Read the model definition and answer for the solid it produces. Units are mm, in the model's axes. A direction names the side the tool comes from. Give positions to 0.01 mm unless a question says otherwise; leave off trailing zeros. Write each loop counter-clockwise with the first axis right and the second up, starting at its lowest first coordinate (ties: lowest second). Pieces come first, ordered by that corner, then holes.
```python
from build123d import *

# Parameters (mm, degrees)
SKETCH_1_W          = 10
SKETCH_1_H          = 10
SKETCH_1_W_2        = 8
SKETCH_1_H_2        = 8
EXTRUDE_1_DEPTH     = 327
SKETCH_2_R          = 2.1
CUT_EXTRUDE_1_DEPTH = 328.191075673
SKETCH_3_R          = 2.1
CUT_EXTRUDE_2_DEPTH = 328.191075673
SKETCH_4_R          = 2.1
CUT_EXTRUDE_3_DEPTH = 328.191075673


with BuildPart() as part:
    # ｽｹｯﾁ1 → 押し出し-薄板1 (new body)
    with BuildSketch(Plane(origin=(0, 0, 0), x_dir=(1, 0, 0), z_dir=(0, 1, 0))):
        Rectangle(SKETCH_1_W, SKETCH_1_H)
        Rectangle(SKETCH_1_W_2, SKETCH_1_H_2, mode=Mode.SUBTRACT)
    extrude(amount=EXTRUDE_1_DEPTH)

    # ｽｹｯﾁ2 → ｶｯﾄ - 押し出し1 (cut, through all)
    with BuildSketch(Plane(origin=(5, 0, 0), x_dir=(0, 0, -1), z_dir=(1, 0, 0))):
        with Locations((0, 322)):
            Circle(SKETCH_2_R)
        with Locations((0, 5)):
            Circle(SKETCH_2_R)
    extrude(amount=-CUT_EXTRUDE_1_DEPTH, mode=Mode.SUBTRACT)

    # ｽｹｯﾁ3 → ｶｯﾄ - 押し出し2 (cut, through all)
    with BuildSketch(Plane(origin=(0, 0, -5), x_dir=(-1, 0, 0), z_dir=(0, 0, -1))):
        with Locations((0, 130)):
            Circle(SKETCH_3_R)
        with Locations((0, 75)):
            Circle(SKETCH_3_R)
        with Locations((0, 47)):
            Circle(SKETCH_3_R)
        with Locations((0, 25)):
            Circle(SKETCH_3_R)
    extrude(amount=-CUT_EXTRUDE_2_DEPTH, mode=Mode.SUBTRACT)

    # ｽｹｯﾁ4 → ｶｯﾄ - 押し出し3 (cut, through all)
    with BuildSketch(Plane.XY.offset(5)):
        with Locations((0, 192)):
            Circle(SKETCH_4_R)
        with Locations((0, 227)):
            Circle(SKETCH_4_R)
    extrude(amount=-CUT_EXTRUDE_3_DEPTH, mode=Mode.SUBTRACT)


solid = part.part
```
Item 1: Find the intervals of material crossed by line 1 along Y through (x, z) = (4.25, 0); line 2 along X through (y, z) = (15.5, 3.25), in increasing order.
Result set:
line 1: y = 0 to 2.9, 7.1 to 319.9, 324.1 to 327
line 2: x = -5 to -4, 4 to 5
Item 2: Section A-A (z = 0) is taken. Write down the section's boundary in (x, y).
Result set:
outline: (-5, 0) - (-4, 0) - (-4, 2.9) - (-5, 2.9) - close; (-5, 7.1) - (-4, 7.1) - (-4, 319.9) - (-5, 319.9) - close; (-5, 324.1) - (-4, 324.1) - (-4, 327) - (-5, 327) - close; (4, 0) - (5, 0) - (5, 2.9) - (4, 2.9) - close; (4, 7.1) - (5, 7.1) - (5, 319.9) - (4, 319.9) - close; (4, 324.1) - (5, 324.1) - (5, 327) - (4, 327) - close
Item 3: Section B-B (y = 306.5) is taken. Write down the section's boundary in (x, z).
Result set:
outline: (-5, -5) - (5, -5) - (5, 5) - (-5, 5) - close; hole (-4, -4) - (4, -4) - (4, 4) - (-4, 4) - close
Item 4: This flat-tipped pin is pushed along its axis until it touches: pin 1 Ø1.5 at (x, z) = (-3, 3) entering from +Y. Where does it stop, or does it pass through?
Result set:
pin 1: passes through
Item 5: Section C-C (x = 0) is taken. Give the number of separate pieces and of enclosed holes in the cut face, and give its area (3 significant figures).
Result set:
separate pieces: 14
enclosed holes: 0
area: 604 mm2
Item 6: Which of the six approach directions +Z, -Z, +X, -X, +Y, -Y give full straight-line access (tool end or side, diameter ignored) to faces 1 (the flat face through (5, 161, 0)), 2 (the flat face through (-4, 161, 0))?
Result set:
face 1: +Z, -Z, +X, +Y, -Y
face 2: +Y, -Y
Item 7: Determine the mould class of faces 3 (the flat face through (0, 161, 4)), 4 (the flat face through (4, 161, 0)), 5 (the flat face through (0, 161, 5)), 6 (the flat face through (-4.5, 0, -0.1)) for opening direction Z: pulls with the +Z half, pulls with the -Z half, needs draft (parallel to the pull), parting line crosses it, or undercut.
Result set:
face 3: undercut
face 4: undercut
face 5: pulls with the +Z half
face 6: needs draft
